Verification items for the finished model (mm, model axes). Give positions to 0.01 mm unless a question says otherwise; leave off trailing zeros. Write each loop counter-clockwise with the first axis right and the second up, starting at its lowest first coordinate (ties: lowest second). Pieces come first, ordered by that corner, then holes.
from build123d import *

# Parameters (mm, degrees)
F0_R     = 39.28888
F1_DEPTH = 50.8
F2_R     = 19.028102
F3_DEPTH = 25
F4_DEPTH = 71


with BuildPart() as f1:
    # F0 (on Front) → F1 (new body)
    with BuildSketch(Plane.XZ):
        with Locations((-10.59674, 24.287323)):
            Circle(F0_R)
    extrude(amount=-F1_DEPTH)

    # F2 (on face) → F3 (cut)
    with BuildSketch(Plane.XZ):
        with Locations((-11.212225, 20.733649)):
            Circle(F2_R)
    extrude(amount=F3_DEPTH, mode=Mode.SUBTRACT)

    # F2 (on face) → F4 (cut)
    with BuildSketch(Plane.XZ):
        with Locations((-11.212225, 20.733649)):
            Circle(F2_R)
    extrude(amount=-F4_DEPTH, mode=Mode.SUBTRACT)


solid = f1.part
Item 1: Depth check by flat-ended pin: pin 1 (1 mm diameter, centred on x = -41, y = 28.5, fed in from +Z); pin 2 (6 mm diameter, centred on x = 16, y = 37, fed in from +Z); pin 3 (2 mm diameter, centred on y = 44, z = -5, fed in from +X). Enter the tip coordinate at first touch or a pass-through.
Answer key:
pin 1: stops at z = 49.77
pin 2: stops at z = 55.7
pin 3: stops at x = 16.67
Item 2: Sectioned sample at A-A on x = 0.5. Record the cut outline in (y, z), then the cut area to 3 significant figures.
Answer key:
outline: (0, -13.4) - (50.8, -13.4) - (50.8, 5.74) - (0, 5.74) - close; (0, 35.73) - (50.8, 35.73) - (50.8, 61.98) - (0, 61.98) - close
area: 2,310 mm2
Item 3: Sectioned sample at C-C on y = 23.5. Record the cut outline in (x, z), then the cut area to 3 significant figures.
Answer key:
outline: circle Ø78.58 at (-10.6, 24.29); hole circle Ø38.06 at (-11.21, 20.73)
area: 3,710 mm2
Item 4: Scan lines: line 1 along X through (y, z) = (2.5, 28.5); line 2 along Z through (x, y) = (-3.5, 16); line 3 along Z through (x, y) = (-18, 25). Record each from-to range of solid material in increasing order.
Answer key:
line 1: x = -49.66 to -28.58, 6.16 to 28.47
line 2: z = -14.36 to 3.34, 38.13 to 62.93
line 3: z = -14.3 to 2.96, 38.51 to 62.87
Item 5: Sectioned sample at B-B on z = 28.5. Record the cut outline in (x, y).
Answer key:
outline: (-49.66, 0) - (-28.58, 0) - (-28.58, 50.8) - (-49.66, 50.8) - close; (6.16, 0) - (28.47, 0) - (28.47, 50.8) - (6.16, 50.8) - close
Item 6: Sectioned sample at D-D on z = 44. Record the cut outline in (x, y).
Answer key:
outline: (-44.58, 0) - (23.39, 0) - (23.39, 50.8) - (-44.58, 50.8) - close
Item 7: Release check for a two-part mould opening along Z. For faces 1 (the face through (-11, 50.8, 42)), 2 (the face through (-15.711, 25.044, 63.242)), 3 (the face through (-30.22, 25.04, 21.57)) record: released by +Z, released by -Z, zero draft, split by the parting line, or undercut.
Answer key:
face 1: zero draft
face 2: split by the parting line
face 3: undercut
